```python
from build123d import *

# Parameters (mm, degrees)
F0_R     = 1.75
F1_DEPTH = 4


with BuildPart() as f1:
    # F0 (on Top) → F1 (new body)
    with BuildSketch(Plane.XY):
        with BuildLine():
            Line((6.0892546755, -33.3552707336), (11.3925555344, -28.0519698747))
            Line((11.3925555344, -28.0519698747), (-9.3547162967, -7.3046980436))
            Line((-9.3547162967, -7.3046980436), (-55.7825886783, 39.1231743381))
            ThreePointArc((-55.7825886783, 39.1231743381), (-58.8891903961, 36.7393949991), (-62.5069047196, 35.2408886615))
            Line((-62.5069047196, 35.2408886615), (-53.2885795254, 26.0225634673))
            Line((-53.2885795254, 26.0225634673), (6.0892546755, -33.3552707336))
        make_face()
        with BuildLine():
            Line((-9.3547162967, -7.3046980436), (11.3925555344, -28.0519698747))
            Line((11.3925555344, -28.0519698747), (16.6958563933, -22.7486690158))
            Line((16.6958563933, -22.7486690158), (-42.6819778076, 36.6291651851))
            add(Edge.make_bspline(
                [(-42.6819778076, 36.6291651851), (-45.2945511903, 39.5061130095), (-50.0695074398, 44.7616576166), (-51.1430333829, 50.0297724966), (-51.6312848813, 52.4138447612)],
                knots=[0, 0, 0, 0, 0.5473526332, 1, 1, 1, 1], degree=3))
            ThreePointArc((-51.6312848813, 52.4138447612), (-51.4017631208, 49.1157535279), (-51.9003030018, 45.8474903793))
            ThreePointArc((-51.9003030018, 45.8474903793), (-53.3988093394, 42.2297760559), (-55.7825886783, 39.1231743381))
            Line((-55.7825886783, 39.1231743381), (-9.3547162967, -7.3046980436))
        make_face()
        with BuildLine():
            ThreePointArc((-62.5069047196, 35.2408886615), (-58.8891903961, 36.7393949991), (-55.7825886783, 39.1231743381))
            ThreePointArc((-55.7825886783, 39.1231743381), (-53.3988093394, 42.2297760559), (-51.9003030018, 45.8474903793))
            ThreePointArc((-51.9003030018, 45.8474903793), (-51.4017631208, 49.1157535279), (-51.6312848813, 52.4138447612))
            ThreePointArc((-51.6312848813, 52.4138447612), (-51.9458010107, 53.7780476698), (-52.3861331822, 55.1069861748))
            add(Edge.make_bspline(
                [(-52.3861331822, 55.1069861748), (-53.6051347333, 55.1308330266), (-56.7515994276, 55.1918775104), (-59.3237157089, 60.4625666695), (-60.9000344454, 63.6893307389)],
                knots=[0, 0, 0, 0, 0.387493123, 1, 1, 1, 1], degree=3))
            ThreePointArc((-60.9000344454, 63.6893307389), (-66.2678346698, 64.7292851408), (-71.6517589086, 63.7763191413))
            add(Edge.make_bspline(
                [(-80.3976496024, 55.0928974107), (-78.8782096295, 56.1643689504), (-75.6891919016, 58.3945745707), (-73.0396610336, 61.9384087083), (-71.6517589086, 63.7763191413)],
                knots=[0, 0, 0, 0, 0.4784709271, 1, 1, 1, 1], degree=3))
            ThreePointArc((-80.3976496024, 55.0928974107), (-81.3784942248, 50.296142309), (-80.7624173443, 45.4390480176))
            add(Edge.make_bspline(
                [(-72.4758721042, 36.0202061945), (-72.6700492153, 37.3502311658), (-73.1313035357, 40.642383964), (-77.9288722558, 43.6485061475), (-80.7624173443, 45.4390480176)],
                knots=[0, 0, 0, 0, 0.4064160365, 1, 1, 1, 1], degree=3))
            ThreePointArc((-72.4758721042, 36.0202061945), (-70.8057804399, 35.3947234788), (-69.0732591015, 34.971870541))
            ThreePointArc((-69.0732591015, 34.971870541), (-65.7751678682, 34.7423487805), (-62.5069047196, 35.2408886615))
        make_face()
        with Locations((-74.3891903961, 49.7297760559)):
            Circle(F0_R, mode=Mode.SUBTRACT)
        with BuildLine():
            ThreePointArc((-64.6391903961, 40.2297760559), (-64.9694713976, 39.2065957368), (-65.8356452136, 38.5696291555))
            ThreePointArc((-65.8356452136, 38.5696291555), (-67.6266272632, 38.9923391888), (-68.0493372965, 40.7833212384))
            ThreePointArc((-68.0493372965, 40.7833212384), (-67.4123707152, 41.6494950544), (-66.3891903961, 41.9797760559))
            ThreePointArc((-66.3891903961, 41.9797760559), (-65.1517535291, 41.4672129229), (-64.6391903961, 40.2297760559))
        make_face(mode=Mode.SUBTRACT)
        with BuildLine():
            ThreePointArc((-62.3891903961, 49.7297760559), (-62.6936722661, 48.1990423264), (-63.5607632714, 46.9013489311))
            ThreePointArc((-63.5607632714, 46.9013489311), (-70.0847085262, 51.2605097853), (-62.3891903961, 49.7297760559))
        make_face(mode=Mode.SUBTRACT)
        with BuildLine():
            ThreePointArc((-60.1391903961, 49.7297760559), (-58.3891903961, 51.4797760559), (-56.6391903961, 49.7297760559))
            ThreePointArc((-56.6391903961, 49.7297760559), (-58.3891903961, 47.9797760559), (-60.1391903961, 49.7297760559))
        make_face(mode=Mode.SUBTRACT)
        with BuildLine():
            ThreePointArc((-66.3891903961, 57.4797760559), (-67.6266272632, 60.4672129229), (-64.6391903961, 59.2297760559))
            ThreePointArc((-64.6391903961, 59.2297760559), (-65.1517535291, 57.9923391888), (-66.3891903961, 57.4797760559))
        make_face(mode=Mode.SUBTRACT)
        with BuildLine():
            add(Edge.make_bspline(
                [(-53.2885795254, 26.0225634673), (-56.1655273498, 28.63513685), (-61.4210719568, 33.4100930995), (-66.6891868368, 34.4836190426), (-69.0732591015, 34.971870541)],
                knots=[0, 0, 0, 0, 0.5473526332, 1, 1, 1, 1], degree=3))
            Line((-53.2885795254, 26.0225634673), (-62.5069047196, 35.2408886615))
            ThreePointArc((-62.5069047196, 35.2408886615), (-65.7751678682, 34.7423487805), (-69.0732591015, 34.971870541))
        make_face()
    extrude(amount=F1_DEPTH)


solid = f1.part
```
Here's how the part is built. I have some questions about the finished solid (model axes, mm). Round coordinates to 2 decimals unless told otherwise and drop trailing zeros. Order: outer loops, then holes, each group sorted by start corner. A loop starts at its lowest first (then second) coordinate and runs counter-clockwise, first axis right, second up. Notation, with made-up numbers: M -25,-20 L -1,-20 A21 ccw -1,-10 Z; hole C 31.25,-38.5 d5. An arc over 180 degrees is marked long. Answer in a Markdown table with one row per item.
Item 1: Imagine slicing it at A-A, the plane z = 2.1. State how many separate pieces and enclosed holes the cut face has, and give its area (3 significant figures).
A:
| item | result |
|---|---|
| separate pieces | 1 |
| enclosed holes | 5 |
| area | 2,010 mm2 |
Item 2: Thinking about a two-plate mould opening in X: for faces 1 (the face through (-76.137, 49.807, 1.972)), 2 (the face through (-59.78, 50.79, 1.97)), 3 (the face through (-66.19, 64.73, 1.97)), 4 (the face through (-24.015, -3.251, 1.972)), which applies, +X half, -X half, draft (parallel to the pull), parting line (faces both ways), or undercut?
A:
| item | result |
|---|---|
| face 1 | undercut |
| face 2 | undercut |
| face 3 | parting line |
| face 4 | -X half |
Item 3: If I drill on L1, parallel to X at y = 47, z = 1.15; L2, parallel to X at y = -1, z = 3.6; L3, parallel to Y at x = 9, z = 3.1, over which ranges is the centre line in solid material (lowest first)? Write a range as from..to.
A:
| item | result |
|---|---|
| L1 | x = -81.14..-69.31, -63.47..-50.2 |
| L2 | x = -26.27..-5.05 |
| L3 | y = -30.44..-15.05 |
Item 4: I'm going to push flat-ended pins straight in: pin 1 (13 mm diameter, centred on x = -66.39, y = 49.73, fed in from +Z); pin 2 (5 mm diameter, centred on x = -27.5, y = 26.5, fed in from -Z); pin 3 (1.5 mm diameter, centred on x = -22.5, z = 2, fed in from -Y). Where does each tip first touch, or does it pass through?
A:
| item | result |
|---|---|
| pin 1 | stops at z = 4 |
| pin 2 | passes through |
| pin 3 | stops at y = -5.52 |
Item 5: Imagine slicing it at C-C, the plane y = 11. Write out the boundary of the cut face in (x, z), and give its area (3 significant figures).
A:
| item | result |
|---|---|
| outline | M -38.27,0 L -17.05,0 L -17.05,4 L -38.27,4 Z |
| area | 84.9 mm2 |
Item 6: Imagine slicing it at B-B, the plane x = -21.5. Write out the boundary of the cut face in (y, z).
A:
| item | result |
|---|---|
| outline | M -5.77,0 L 15.45,0 L 15.45,4 L -5.77,4 Z |
